from build123d import *

# Parameters (mm, degrees)
F0_W     = 51.462281
F0_H     = 56.140669
F1_DEPTH = 25.4
F2_R     = 12.7
F3_DEPTH = 25.4
F4_W     = 30.184469
F4_H     = 9.87075
F5_DEPTH = 25.4


with BuildPart() as f1:
    # F0 (on Front) → F1 (new body)
    with BuildSketch(Plane.XZ):
        with Locations((25.73114, 28.070334)):
            Rectangle(F0_W, F0_H)
    extrude(amount=F1_DEPTH)

    # F2 (on face) → F3 (cut)
    with BuildSketch(Plane.XZ.offset(25.4)):
        with Locations((25.77888, 27.688427)):
            Circle(F2_R)
    extrude(amount=-F3_DEPTH, mode=Mode.SUBTRACT)

    # F4 (on face) → F5 (cut)
    with BuildSketch(Plane.XY.offset(56.140669)):
        with Locations((23.83924, -11.24981)):
            Rectangle(F4_W, F4_H)
    extrude(amount=-F5_DEPTH, mode=Mode.SUBTRACT)


solid = f1.part
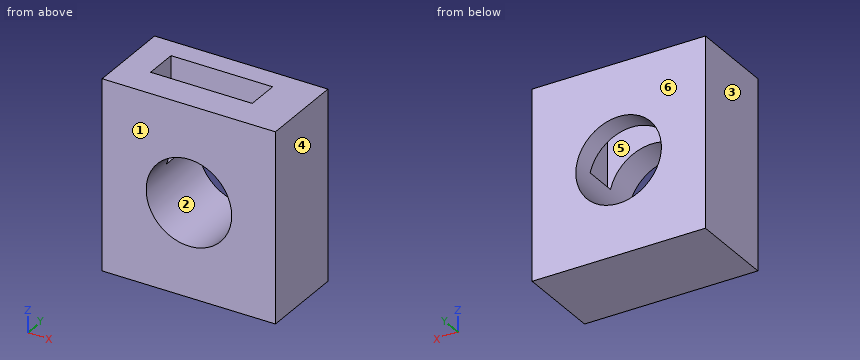
Design review of the part built by this model. Coordinates are the model's own, in mm. Face numbers are marked on the shaded views. A direction names the side the tool comes from. Coordinates: 2 decimals unless noted, no trailing zeros. Order: outer loops, then holes, each group sorted by start corner. A loop starts at its lowest first (then second) coordinate and runs counter-clockwise, first axis right, second up.
Item 1: For pin 1 Ø6 at (x, y) = (27.5, -10.5) entering from +Z; pin 2 Ø5 at (x, y) = (12, -11) entering from +Z; pin 3 Ø12.5 at (x, z) = (21, 39.5) entering from +Y, all flat-tipped, find the tip position at first contact; note any pin that passes through.
Item 2: Take a section at D-D, the plane x = 19. Write out the cut boundary in (y, z), then the cut area to 3 significant figures.
Item 3: For line 1 (X direction, y = -15.5, z = 40.5); line 2 (Y direction, x = 16, z = 42); line 3 (Z direction, x = 35.5, y = -16.5), list the stretches that pass through material, from the lowest coordinate up.
Item 4: Take a section at A-A, the plane x = 9.5. Write out the cut boundary in (y, z), then the cut area to 3 significant figures.
Item 5: For the marked faces 5 and 6, list the 3-axis set-ups (+Z, -Z, +X, -X, +Y, -Y) from which the entire face can be reached by the end or side of a thin tool; tool diameter is ignored.
Item 6: The part is to be moulded in two halves that separate along X. For the marked faces 1, 2, 3 and 4, say which applies: pulls with the +X half, pulls with the -X half, needs draft (parallel to the pull), parting line crosses it, or undercut.
Item 7: Take a section at C-C, the plane y = -15.5. Write out the cut boundary in (x, z), then the cut area to 3 significant figures.
Item 8: Take a section at B-B, the plane z = 16. Write out the cut boundary in (x, y), then the cut area to 3 significant figures.
The answers:
1. pin 1: stops at z = 15.9
1. pin 2: stops at z = 30.74
1. pin 3: stops at y = 0
2. outline: (-25.4, 0) - (0, 0) - (0, 16.95) - (-25.4, 16.95) - close; (-25.4, 38.43) - (-16.19, 38.43) - (-16.19, 56.14) - (-25.4, 56.14) - close; (-6.31, 38.43) - (0, 38.43) - (0, 56.14) - (-6.31, 56.14) - close
2. area: 706 mm2
3. line 1: x = 0 to 8.75, 38.93 to 51.46
3. line 2: y = -25.4 to -16.19, -6.31 to 0
3. line 3: z = 0 to 19.52, 35.86 to 56.14
4. outline: (-25.4, 0) - (0, 0) - (0, 56.14) - (-6.31, 56.14) - (-6.31, 30.74) - (-16.19, 30.74) - (-16.19, 56.14) - (-25.4, 56.14) - close
4. area: 1,180 mm2
5. face 5: +Z
5. face 6: +Z, -Z, +X, -X, +Y
6. face 1: needs draft
6. face 2: undercut
6. face 3: pulls with the -X half
6. face 4: pulls with the +X half
7. outline: (0, 0) - (51.46, 0) - (51.46, 56.14) - (38.93, 56.14) - (38.93, 30.74) - (38.11, 30.74) arc R12.7 cw (long way) to (13.45, 30.74) - (8.75, 30.74) - (8.75, 56.14) - (0, 56.14) - close
7. area: 1,790 mm2
8. outline: (0, -25.4) - (20.81, -25.4) - (20.81, 0) - (0, 0) - close; (30.75, -25.4) - (51.46, -25.4) - (51.46, 0) - (30.75, 0) - close
8. area: 1,050 mm2
